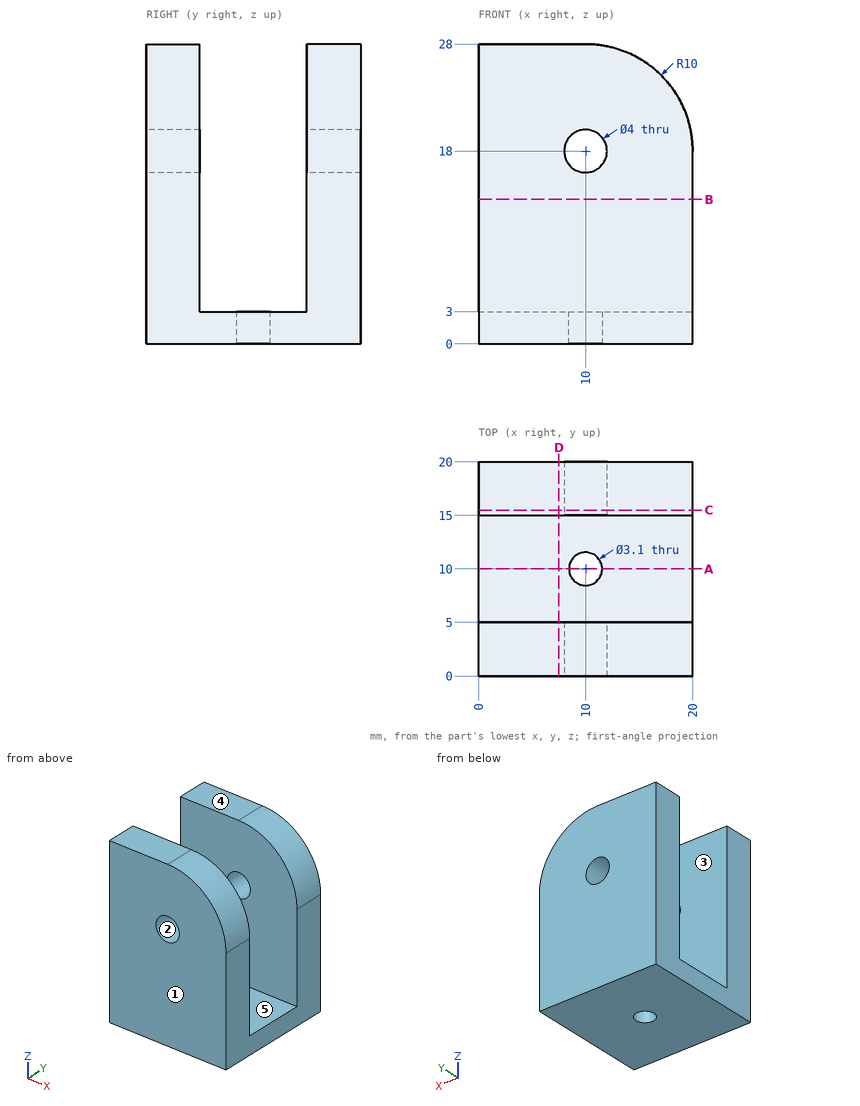
Check sheet for the drawn part. Datum: minimum x, y, z corner. Units: mm. A direction names the side the tool comes from. Round coordinates to 2 decimals unless told otherwise and drop trailing zeros. Loops run counter-clockwise (first coordinate to the right, second up) from the corner with the lowest first, then second, coordinate; pieces in that order, holes last. Notation, with made-up numbers: M -5,4 L 14,4 A20 cw 14,35 Z; hole C -6.75,-20.5 d1. An arc over 180 degrees is marked long. One line per question, with ' | ' between items. Start each with the question number.
Item 1: Set-up check for the marked faces 4 and 5: record each of +Z, -Z, +X, -X, +Y, -Y from which the full face is reachable in a straight line by a thin tool's end or side.
Item 2: Section check B-B (z = 13.5). Record the boundary of the cut face in (x, y).
Item 3: Release check for a two-part mould opening along Y. For the marked faces 1, 2 and 3 record: released by +Y, released by -Y, zero draft, split by the parting line, or undercut.
Item 4: Gauge pin test, flat ends, axial feed: pin 1 Ø8 at (x, z) = (9.5, 11) entering from -Y; pin 2 Ø6 at (x, y) = (14, 2) entering from +Z; pin 3 Ø8 at (x, y) = (6, 9.5) entering from +Z. Record the tip position at first contact, or that the pin passes through.
Item 5: Scan lines: probe 1 along Y at (x, z) = (8, 20.5); probe 2 along Z at (x, y) = (10, 18.4); probe 3 along Y at (x, z) = (10, 2). Record each from-to range of solid material in increasing order.
Item 6: Section check D-D (x = 7.5). Record the boundary of the cut face in (y, z).
Item 7: Section check C-C (y = 15.5). Record the boundary of the cut face in (x, z), and give its area (3 significant figures).
Item 8: Section check A-A (y = 10). Record the boundary of the cut face in (x, z), and give its area (3 significant figures).
Worked out:
1) face 4: +Z, +X, -X, +Y, -Y | face 5: +Z, +X, -X
2) outline: M 0,0 L 20,0 L 20,5 L 0,5 Z; M 0,15 L 20,15 L 20,20 L 0,20 Z
3) face 1: released by -Y | face 2: zero draft | face 3: undercut
4) pin 1: y = 0 | pin 2: z = 27.95 | pin 3: z = 3
5) probe 1: 0 to 5, 15 to 20 | probe 2: 0 to 16, 20 to 28 | probe 3: 0 to 8.45, 11.55 to 20
6) outline: M 0,0 L 20,0 L 20,28 L 15,28 L 15,3 L 5,3 L 5,28 L 0,28 Z
7) outline: M 0,0 L 20,0 L 20,18 A10 ccw 10,28 L 0,28 Z; hole C 10,18 d4 | area: 526 mm^2
8) outline: M 0,0 L 8.45,0 L 8.45,3 L 0,3 Z; M 11.55,0 L 20,0 L 20,3 L 11.55,3 Z | area: 50.7 mm^2
